```python
from build123d import *

# Parameters (mm, degrees)
BOSS_EXTRU_1_DEPTH      = 30
ENL_V_MAT_EXTRU_1_DEPTH = 40
CHANFREIN1_SIZE         = 5
CHANFREIN1_SIZE_2       = 4.485876758
CHANFREIN1_SIZE_3       = 4.444390394


with BuildPart() as part:
    # Esquisse1 → Boss.-Extru.1 (new body)
    with BuildSketch(Plane.XY):
        Polygon((-20.683192831, -25.589578536), (0, 32.410421464), (20.216807169, -25.589578536), (25.216807169, -25.589578536), (0.052428935, 46.604508561), (-25.692471491, -25.589578536), align=None)
    extrude(amount=BOSS_EXTRU_1_DEPTH)

    # Esquisse2 → Enlèv. mat.-Extru.1 (cut, symmetric)
    with BuildSketch(Plane(origin=(0, 0, 0), x_dir=(0, 0, -1), z_dir=(1, 0, 0))):
        Polygon((-30, 46.604508561), (-7.091444924, -16.336229224), (-30, -16.777180943), align=None)
    extrude(amount=ENL_V_MAT_EXTRU_1_DEPTH, both=True, mode=Mode.SUBTRACT)

    # Chanfrein1
    # the kernel refuses this chamfer: 5, 4.485876758, 4.444390394 mm, written as the material it takes off along each edge
    with BuildSketch(Plane(origin=(-22.303983799, -16.087550115, -5.828062673), x_dir=(0.9997543804703944, 0.020937821677919046, 0.0072654217800036), z_dir=(-0.00686265654519205, -0.019244324745599332, 0.9997912581685382))) as chanfrein1_piece_1_section:
        Polygon((CHANFREIN1_SIZE * 0.999777923546, -CHANFREIN1_SIZE * 0.0210737654663), (-CHANFREIN1_SIZE_2 * 0.35560163891, -CHANFREIN1_SIZE_2 * 0.934637616571), (0, 0), align=None)
    chanfrein1_piece_1 = extrude(amount=48.757748051, mode=Mode.PRIVATE)
    chanfrein1_piece_1 = split(chanfrein1_piece_1, bisect_by=Plane(origin=(-21.319692557, -14.185364149, 7.874295789), z_dir=(0, -0.3420201433256631, 0.9396926207859105)), keep=Keep.TOP, mode=Mode.PRIVATE)
    add(chanfrein1_piece_1, mode=Mode.SUBTRACT)
    with BuildSketch(Plane(origin=(22.231789239, -17.025860313, 42.919521162), x_dir=(0.35409216493463397, -0.9349886052835225, -0.0203726954985718), z_dir=(-0.006707917430774409, 0.01924434495210566, -0.9997923079475588))) as chanfrein1_piece_2_section:
        Polygon((CHANFREIN1_SIZE_3 * 0.999645713908, CHANFREIN1_SIZE_3 * 0.0266166655786), (-CHANFREIN1_SIZE * 0.354100131597, CHANFREIN1_SIZE * 0.935207515369), (0, 0), align=None)
    chanfrein1_piece_2 = extrude(amount=48.757723993, mode=Mode.PRIVATE)
    chanfrein1_piece_2 = split(chanfrein1_piece_2, bisect_by=Plane(origin=(20.901821142, -14.176256403, 7.877610737), z_dir=(0, -0.3420201433256631, 0.9396926207859105)), keep=Keep.TOP, mode=Mode.PRIVATE)
    add(chanfrein1_piece_2, mode=Mode.SUBTRACT)


solid = part.part
```
Geometry: final body of the model. Coordinates: model frame, mm. Give positions to 0.01 mm unless a question says otherwise; leave off trailing zeros. Order: outer loops, then holes, each group sorted by start corner. A loop starts at its lowest first (then second) coordinate and runs counter-clockwise, first axis right, second up. Notation, with made-up numbers: M -6.75,52 L 12.25,52 A27 cw 12.25,78 Z; hole C 50,45 d4. An arc over 180 degrees is marked long. Answer as CSV lines item,"result". Start each with the question number.
1) Cut plane B-B (z = 14). State how many separate pieces and enclosed holes the cut face has, then the cut area to 3 significant figures.
2) Cut plane D-D (y = 22.5). Output: boundary loops of the cut face in (x, z).
3) First-contact query: P1, Ø6, axis at x = 3.5, z = 22.5, coming from the -Y side; P2, Ø8, axis at y = 35.5, z = 3.5, coming from the -X side; P3, Ø1, axis at y = 11.5, z = 8, coming from the +X side. Flat tips, straight axial feed; report the tip coordinate or a pass-through.
4) Cut plane C-C (x = 18). Output: boundary loops of the cut face in (y, z).
5) Cut plane A-A (y = 11). Output: boundary loops of the cut face in (x, z).
6) Line query: line 1 (X direction, y = 18, z = 13.5); line 2 (X direction, y = 3, z = 14); line 3 (Z direction, x = 6.5, y = 23.5). Output: solid intervals per line, ascending. Write a range as from..to.
7) Mould query, pull axis X, two halves, no side actions, for faces 1 (the flat face through (-10.49, 3, 8.12)), 2 (the flat face through (-22, -22, 30)), 3 (the flat face through (-12.64, 11.01, 11.46)), 4 (the flat face through (9.967, 3.816, 11.457)). Classes: +X half, -X half, draft (parallel to the pull), parting line (faces both ways), or undercut.
Findings below:
1,separate pieces,"3"
1,enclosed holes,"0"
1,area,"439 mm²"
2,outline,"M -8.54,0 L -3.53,0 L -3.53,21.23 L -8.54,21.23 Z; M 3.45,0 L 8.45,0 L 8.45,21.23 L 3.45,21.23 Z"
3,P1,"stops at y = 18.59"
3,P2,"stops at x = -5.33"
3,P3,"stops at x = 12.46"
4,outline,"M -19.23,0 L -4.89,0 L -4.89,11.26 L -16.99,6.85 L -17.33,30 L -19.23,30 Z"
5,outline,"M -12.64,0 L -7.64,0 L -7.64,17.04 L -12.64,17.04 Z; M 7.46,0 L 12.46,0 L 12.46,17.04 L 7.46,17.04 Z"
6,line 1,"x = -10.15..-5.14, 5.02..10.02"
6,line 2,"x = -15.5..-10.49, 10.25..15.25"
6,line 3,"z = 0..21.59"
7,face 1,"undercut"
7,face 2,"draft"
7,face 3,"-X half"
7,face 4,"undercut"
